```python
from build123d import *

# Parameters (mm, degrees)
F0_R     = 8
F1_DEPTH = 8
F2_R     = 6
F4_R     = 5.5
F6_R     = 1


with BuildPart() as f1:
    # F0 (on Top) → F1 (new body)
    with BuildSketch(Plane.XY):
        Circle(F0_R)
    extrude(amount=F1_DEPTH)

    # F2 (on face) → F5 section 0
    with BuildSketch(Plane.XY.offset(8)):
        Circle(F2_R)
    # F4 (on offset) → F5 section 1
    with BuildSketch(Plane.XY.offset(24)):
        Circle(F4_R)
    loft()

    # F6
    f6_edges = [f1.edges().sort_by_distance(p)[0] for p in [
        (-5.5, 0, 24),
    ]]
    fillet(f6_edges, radius=F6_R)


solid = f1.part
```
Geometry check sheet. Reference: the model listing, model coordinates, mm. A direction names the side the tool comes from. Coordinates: 2 decimals unless noted, no trailing zeros. Order: outer loops, then holes, each group sorted by start corner. A loop starts at its lowest first (then second) coordinate and runs counter-clockwise, first axis right, second up.
Q1. Sectioned sample at B-B on z = 5.5. Record the cut outline in (x, y).
Reply:
outline: circle Ø16 at (0, 0)
Q2. Sectioned sample at C-C on z = 21.75. Record the cut outline in (x, y).
Reply:
outline: circle Ø11.14 at (0, 0)
Q3. Sectioned sample at A-A on x = 0. Record the cut outline in (y, z).
Reply:
outline: (-8, 0) - (8, 0) - (8, 8) - (6, 8) - (5.53, 23.03) arc R1 ccw to (4.53, 24) - (-4.53, 24) arc R1 ccw to (-5.53, 23.03) - (-6, 8) - (-8, 8) - close
Q4. Thickness scan on probe 1 along Z at (x, y) = (3.5, 5.5); probe 2 along X at (y, z) = (-2.25, 7.25); probe 3 along Y at (x, z) = (-4, 9.25). Record the ranges inside material, lowest first.
Reply:
probe 1: z = 0 to 8
probe 2: x = -7.68 to 7.68
probe 3: y = -4.42 to 4.42
Q5. Tool access check on faces 1 (the face through (-2, 6, 8)), 2 (the face through (-1.73, -7.81, 3.94)). Record the directions out of +Z, -Z, +X, -X, +Y, -Y that give a thin tool (end or side, any length) a straight path to the whole face; none if there is none.
Reply:
face 1: +Z
face 2: +Z, -Z
Q6. Sectioned sample at D-D on x = 7. Record the cut outline in (y, z), and give its area (3 significant figures).
Reply:
outline: (-3.87, 0) - (3.87, 0) - (3.87, 8) - (-3.87, 8) - close
area: 62.0 mm2
Q7. Depth check by flat-ended pin: pin 1 Ø5 at (y, z) = (5.5, 17.5) entering from -X; pin 2 Ø8 at (x, z) = (-3.5, 18) entering from +Y; pin 3 Ø1.5 at (x, y) = (4.5, 4) entering from +Z. Enter the tip coordinate at first touch or a pass-through.
Reply:
pin 1: stops at x = -4.85
pin 2: stops at y = 5.75
pin 3: stops at z = 23.67
